Verification items for this drawing (mm, ordinates from the low corner). A direction names the side the tool comes from. Coordinates: 2 decimals unless noted, no trailing zeros. Order: outer loops, then holes, each group sorted by start corner. A loop starts at its lowest first (then second) coordinate and runs counter-clockwise, first axis right, second up. Notation, with made-up numbers: (-18, 64.25) -> (-13, 64.25) arc R23 cw to (-13, 89.25) -> close; hole circle Ø7 at (30, 72.25). An arc over 180 degrees is marked (long way). Write each question's results on one line, items separated by ' | '. Start each with the question number.
(1) Cross-section at C-C on y = 7.1. Enter the section's corners in (x, z) (3 decimals), and give its area (3 significant figures).
(2) Thickness scan on probe 1 along Y at (x, z) = (0.55, 3.6) (3 decimals); probe 2 along X at (y, z) = (0.55, 3.6); probe 3 along X at (y, z) = (0.2, 3.6). Record the ranges inside material, lowest first. Write a range as [from, to].
(3) Cross-section at B-B on x = 5.4. Enter the section's corners in (y, z).
(4) Go/stop test with flat-tipped pins: pin 1 (1.5 mm diameter, centred on x = 3, z = 5.5, fed in from +Y); pin 2 (1.5 mm diameter, centred on y = 8.5, z = 5, fed in from +X). Record where each tip stops, or that it passes through.
(5) Cross-section at D-D on z = 1.5. Enter the section's corners in (x, y), and give its area (3 significant figures).
(6) Cross-section at A-A on z = 3.6. Enter the section's corners in (x, y) (3 decimals).
(7) Set-up check for the marked faces 1 and 2: record each of +Z, -Z, +X, -X, +Y, -Y from which the full face is reachable in a straight line by a thin tool's end or side.
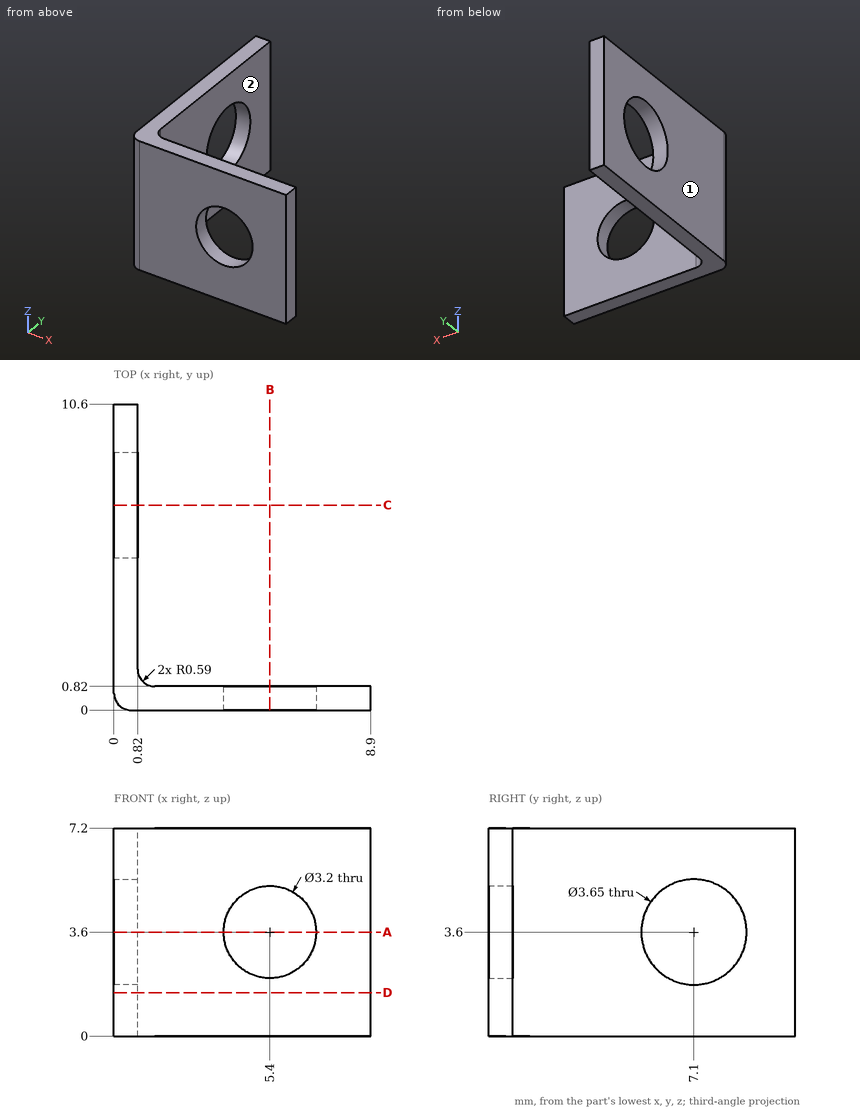
Results are:
1) outline: (0, 0) -> (0.82, 0) -> (0.82, 1.775) -> (0, 1.775) -> close; (0, 5.425) -> (0.82, 5.425) -> (0.82, 7.2) -> (0, 7.2) -> close | area: 2.91 mm2
2) probe 1: y = [0.001, 5.275], [8.925, 10.6] | probe 2: x = [0, 3.8], [7, 8.9] | probe 3: x = [0.15, 3.8], [7, 8.9]
3) outline: (0, 0) -> (0.82, 0) -> (0.82, 2) -> (0, 2) -> close; (0, 5.2) -> (0.82, 5.2) -> (0.82, 7.2) -> (0, 7.2) -> close
4) pin 1: stops at y = 0.82 | pin 2: stops at x = 0.82
5) outline: (0, 0.59) arc R0.59 ccw to (0.59, 0) -> (8.9, 0) -> (8.9, 0.82) -> (1.41, 0.82) arc R0.59 cw to (0.82, 1.41) -> (0.82, 10.6) -> (0, 10.6) -> close | area: 15.3 mm2
6) outline: (0, 0.59) arc R0.59 ccw to (0.59, 0) -> (3.8, 0) -> (3.8, 0.82) -> (1.41, 0.82) arc R0.59 cw to (0.82, 1.41) -> (0.82, 5.275) -> (0, 5.275) -> close; (0, 8.925) -> (0.82, 8.925) -> (0.82, 10.6) -> (0, 10.6) -> close; (7, 0) -> (8.9, 0) -> (8.9, 0.82) -> (7, 0.82) -> close
7) face 1: +Z, -Z, -X, +Y, -Y | face 2: +Z, -Z, +X, +Y
